from build123d import *

# Parameters (mm, degrees)
SKETCH_1_W      = 2
SKETCH_1_H      = 5
EXTRUDE_1_DEPTH = 2
FILLET_1_R      = 10


with BuildPart() as part:
    # 草图1 → 凸台-拉伸1 (new body)
    with BuildSketch(Plane(origin=(0, 0, 0), x_dir=(1, 0, 0), z_dir=(0, 1, 0))):
        with BuildLine():
            Line((10, 0), (0, 0))
            Line((0, 0), (0, -5))
            Line((0, -5), (0, -13.5))
            ThreePointArc((0, -13.5), (1.060660172, -13.939339828), (1.5, -15))
            ThreePointArc((1.5, -15), (1.060660172, -16.060660172), (0, -16.5))
            Line((0, -16.5), (0, -43.5))
            ThreePointArc((0, -43.5), (1.060660172, -43.939339828), (1.5, -45))
            Line((1.5, -45), (2.5, -45))
            Line((2.5, -45), (2.5, -42.5))
            Line((2.5, -42.5), (7.5, -42.5))
            Line((7.5, -42.5), (7.5, -45))
            Line((7.5, -45), (8.5, -45))
            ThreePointArc((8.5, -45), (8.939339828, -43.939339828), (10, -43.5))
            Line((10, -43.5), (10, -16.5))
            ThreePointArc((10, -16.5), (8.5, -15), (10, -13.5))
            Line((10, -13.5), (10, -5))
            Line((10, -5), (10, 0))
        make_face()
        Polygon((2.5, -42.5), (2.5, -45), (5, -45), (7.5, -45), (7.5, -42.5), align=None)
        Polygon((5, -45), (2.5, -45), (2.5, -47.5), (7.5, -47.5), (7.5, -45), align=None)
        with BuildLine():
            Line((2.5, -45), (1.5, -45))
            ThreePointArc((1.5, -45), (1.060660172, -46.060660172), (0, -46.5))
            Line((0, -46.5), (0, -73.5))
            ThreePointArc((0, -73.5), (1.060660172, -73.939339828), (1.5, -75))
            ThreePointArc((1.5, -75), (1.060660172, -76.060660172), (0, -76.5))
            Line((0, -76.5), (0, -85))
            Line((0, -85), (0, -90))
            Line((0, -90), (10, -90))
            Line((10, -90), (10, -85))
            Line((10, -85), (10, -76.5))
            ThreePointArc((10, -76.5), (8.5, -75), (10, -73.5))
            Line((10, -73.5), (10, -46.5))
            ThreePointArc((10, -46.5), (8.939339828, -46.060660172), (8.5, -45))
            Line((8.5, -45), (7.5, -45))
            Line((7.5, -45), (7.5, -47.5))
            Line((7.5, -47.5), (2.5, -47.5))
            Line((2.5, -47.5), (2.5, -45))
        make_face()
        with Locations((11, -87.5)):
            Rectangle(SKETCH_1_W, SKETCH_1_H)
        with Locations((-1, -87.5)):
            Rectangle(SKETCH_1_W, SKETCH_1_H)
        with Locations((11, -2.5)):
            Rectangle(SKETCH_1_W, SKETCH_1_H)
        with Locations((-1, -2.5)):
            Rectangle(SKETCH_1_W, SKETCH_1_H)
    extrude(amount=EXTRUDE_1_DEPTH)

    # 圆角1
    # the kernel refuses this fillet: 10 mm, written as the material it adds along each edge
    with BuildSketch(Plane(origin=(10, 0, 85), x_dir=(0, 0, -1), z_dir=(0, 1, 0)), Plane(origin=(0, 0, 5), x_dir=(0, 0, 1), z_dir=(0, 1, 0))) as fillet_1_piece_1:
        with BuildLine():
            CenterArc((6, -10), FILLET_1_R, 90, 36.869897646)
            Line((0, -2), (0, 0))
            Line((0, 0), (6, 0))
        make_face()
    extrude(amount=2)
    with BuildSketch(Plane(origin=(0, 0, 85), x_dir=(-1, 0, 0), z_dir=(0, 1, 0)), Plane(origin=(10, 0, 5), x_dir=(1, 0, 0), z_dir=(0, 1, 0))) as fillet_1_piece_2:
        with BuildLine():
            CenterArc((10, -6), FILLET_1_R, 143.130102354, 36.869897646)
            Line((0, -6), (0, 0))
            Line((0, 0), (2, 0))
        make_face()
    extrude(amount=2)


solid = part.part
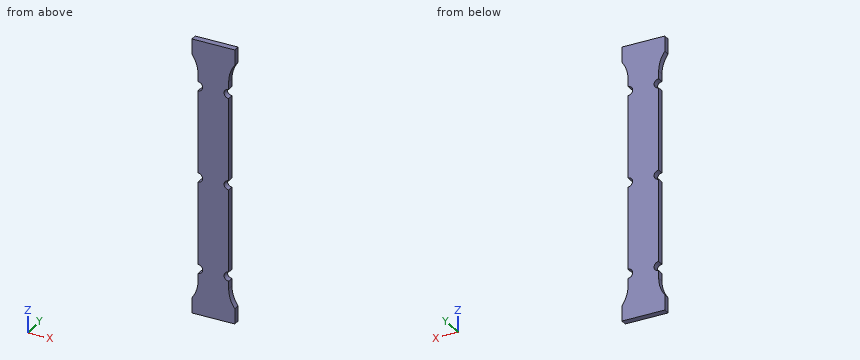
Verification items for the finished model (mm, model axes). Round coordinates to 2 decimals unless told otherwise and drop trailing zeros. Order: outer loops, then holes, each group sorted by start corner. A loop starts at its lowest first (then second) coordinate and runs counter-clockwise, first axis right, second up. Notation, with made-up numbers: (51, -16) -> (81, -16) arc R26 cw to (81, -2) -> close; hole circle Ø9 at (15.5, 88.5). An arc over 180 degrees is marked (long way). Put each result on its own line as item: value.
1) Section check B-B (y = 0.9). Record the cut outline in (x, z), then the cut area to 3 significant figures.
Final values:
outline: (-2, 0) -> (12, 0) -> (12, 5) arc R10 cw to (10, 11) -> (10, 13.5) arc R1.5 cw to (10, 16.5) -> (10, 43.5) arc R1.5 cw to (10, 46.5) -> (10, 73.5) arc R1.5 cw to (10, 76.5) -> (10, 79) arc R10 cw to (12, 85) -> (12, 90) -> (-2, 90) -> (-2, 85) arc R10 cw to (0, 79) -> (0, 76.5) arc R1.5 cw to (0, 73.5) -> (0, 46.5) arc R1.5 cw to (0, 43.5) -> (0, 16.5) arc R1.5 cw to (0, 13.5) -> (0, 11) arc R10 cw to (-2, 5) -> close
area: 934 mm^2
2) Material ranges on line 1 (Z direction, x = 1.25, y = 0.85); line 2 (Z direction, x = 0.25, y = 0.35); line 3 (X direction, y = 0.25, z = 56.5), recorded low to high.
Final values:
line 1: z = 0 to 14.17, 15.83 to 44.17, 45.83 to 74.17, 75.83 to 90
line 2: z = 0 to 13.52, 16.48 to 43.52, 46.48 to 73.52, 76.48 to 90
line 3: x = 0 to 10
3) Section check D-D (z = 58). Record the cut outline in (x, y), then the cut area to 3 significant figures.
Final values:
outline: (0, 0) -> (10, 0) -> (10, 2) -> (0, 2) -> close
area: 20.0 mm^2
4) Section check A-A (x = -1). Record the cut outline in (y, z).
Final values:
outline: (0, 0) -> (2, 0) -> (2, 6.64) -> (0, 6.64) -> close; (0, 83.36) -> (2, 83.36) -> (2, 90) -> (0, 90) -> close
5) Depth check by flat-ended pin: pin 1 (2 mm diameter, centred on x = 6.5, z = 26, fed in from -Y); pin 2 (0.6 mm diameter, centred on y = 1, z = 31, fed in from +X); pin 3 (1 mm diameter, centred on y = 1.5, z = 78, fed in from -X). Enter the tip coordinate at first touch or a pass-through.
Final values:
pin 1: stops at y = 0
pin 2: stops at x = 10
pin 3: stops at x = 0
6) Section check C-C (x = 9.25). Record the cut outline in (y, z).
Final values:
outline: (0, 0) -> (2, 0) -> (2, 13.7) -> (0, 13.7) -> close; (0, 16.3) -> (2, 16.3) -> (2, 43.7) -> (0, 43.7) -> close; (0, 46.3) -> (2, 46.3) -> (2, 73.7) -> (0, 73.7) -> close; (0, 76.3) -> (2, 76.3) -> (2, 90) -> (0, 90) -> close
